Autodesk Inventor part; units mm, degrees
ref_plane "YZ Plane" through (0, 0, 0) normal (1, 0, 0) x (0, 1, 0)
ref_plane "XZ Plane" through (0, 0, 0) normal (0, 1, 0) x (-1, 0, 0)
ref_plane "XY Plane" through (0, 0, 0) normal (0, 0, 1) x (1, 0, 0)
sketch "Sketch1" plane through (0, 0, 0) normal (0, 0, 1) x (1, 0, 0)
  line L0 (-22.5, -30) -> (-22.5, 30)
  line L1 (-22.5, 30) -> (22.5, 30)
  line L2 (22.5, 30) -> (22.5, -30)
  line L3 (22.5, -30) -> (-22.5, -30)
  line L4 (-22.5, -30) -> (22.5, 30) construction
  line L5 (-22.5, 30) -> (22.5, -30) construction
  line L6 (-22.5, 30) -> (-22.5, 22.5)
  line L7 (0, -30) -> (0, -20)
  line L8 (0, -20) -> (-10, -20)
  line L9 (-10, -20) -> (10, -20)
  line L10 (-22.5, 22.5) -> (-10, -20)
  line L11 (22.5, 30) -> (22.5, 22.5)
  line L12 (22.5, 22.5) -> (10, -20)
  arc A0 (-10, -20) -> (10, -20) centre (0, -20) ccw
  point P0 (0, 0)
  dimension "d0" = 60
  dimension "d1" = 45
  dimension "d2" = 7.5
  dimension "d3" = 10
  dimension "d4" = 10
  dimension "d5" = 20
  dimension "d6" = 7.5
extrude "Extrusion1" add sketch "Sketch1" along normal blind 40 contours L0 L1 L2 L12 L9 L8 L10 | A0 L8 L7 | L7 L9 A0
sketch "Sketch2" plane through (0, 0, 0) normal (1, 0, 0) x (0, 1, 0)
  line L0 (30, 0) -> (30, 40)
  line L1 (30, 40) -> (30, 0)
  line L2 (-20, 0) -> (-30, 0)
  line L3 (30, 0) -> (-30, 0)
  line L4 (-30, 0) -> (-30, 1)
  line L5 (-30, 0) -> (-30, 40)
  line L6 (30, 40) -> (-30, 40)
  line L7 (-30, 40) -> (-30, 39)
  line L8 (-30, 39) -> (27.8612, 39)
  line L9 (30, 40) -> (22.5, 40)
  line L10 (-30, 1) -> (27.8612, 1)
  line L11 (27.8612, 1) -> (27.8612, 39)
  line L12 (-30, 39) -> (-30, 1)
  point P0 (0, 0)
  dimension "d9" = 1
  dimension "d10" = 1
extrude "Extrusion2" cut sketch "Sketch2" along normal through all both and the other way through all contours L5 L8 L11 L10
sketch "Sketch3" plane through (0, 0, 40) normal (0, 0, 1) x (1, 0, 0)
  arc A0 (-10, -20) -> (10, -20) centre (0, -20) ccw
  line L0 (10, -20) -> (22.5, 22.5)
  line L1 (22.5, 22.5) -> (22.5, 30)
  line L2 (22.5, 30) -> (-22.5, 30)
  line L3 (-22.5, 30) -> (-22.5, 22.5)
  line L4 (-22.5, 22.5) -> (-10, -20)
  circle A1 centre (0, -25.2901) radius 2.5
  point P0 (0, 0)
  dimension "d13" = 5
extrude "Extrusion3" cut sketch "Sketch3" against normal blind 40 contours A1
sketch "Sketch4" plane through (-22.5, 30, 0) normal (0, 1, 0) x (1, 0, 0)
  line L0 (45, -40) -> (0, -40)
  line L1 (45, 0) -> (0, 0)
  line L2 (0, -40) -> (45, 0) construction
  line L3 (0, 0) -> (0, -40)
  line L4 (0, 0) -> (45, -40) construction
  line L5 (0, -20) -> (45, -20) construction
  circle A0 centre (4.5627, -20) radius 2.5
  point P0 (22.5, 0)
  dimension "d16" = 5
extrude "Extrusion4" cut sketch "Sketch4" against normal blind 10
ref_plane "Work Plane1" through (0, 22.5, 0) normal (1, 0, 0) x (0, 0, -1)
mirror "Mirror1" about plane through (0, 22.5, 0) normal (1, 0, 0) of "Extrusion4"
properties part number "Thin Wheel Mount"
Check sheet for the modelled part. Datum: model origin and axes. Units: mm. A direction names the side the tool comes from. Give positions to 0.01 mm unless a question says otherwise; leave off trailing zeros. Order: outer loops, then holes, each group sorted by start corner. A loop starts at its lowest first (then second) coordinate and runs counter-clockwise, first axis right, second up. Notation, with made-up numbers: M 63,72 L 118,72 A22 cw 118,105 Z; hole C 41,32.25 d8. An arc over 180 degrees is marked long. Answer in a Markdown table with one row per item. Add a question column.
Q1. Gauge pin test, flat end, axial feed: pin 1 Ø5 at (x, z) = (3.5, 31) entering from -Y. Record the tip position at first contact, or that the pin passes through.
Q2. Release check for a two-part mould opening along X. For faces 1 (the flat face through (-22.5, 28.5, 19.9)), 2 (the flat face through (0, 30, 20)), 3 (the cylindrical face through (1.15, -27.51, 39.51)) record: released by +X, released by -X, zero draft, split by the parting line, or undercut.
Q3. Sectioned sample at C-C, the plane x = 19. Record the boundary of the cut face in (y, z).
Q4. Sectioned sample at B-B, the plane x = 0. Record the boundary of the cut face in (y, z), and give its area (3 significant figures).
Q5. Sectioned sample at D-D, the plane y = 11. Record the boundary of the cut face in (x, z), and give its area (3 significant figures).
Q6. Access from +Z, -Z, +X, -X, +Y, -Y to the whole of each face (thin tool, end or side, straight path). Record for faces 4 (the flat face through (0, 5, 39)), 5 (the flat face through (16.34, 1.55, 39.49)).
Q7. Thickness scan on L1, parallel to X at y = 28, z = 20; L2, parallel to Z at x = -7, y = -19.5; L3, parallel to Y at x = 0, z = 0.55. Record the ranges inside material, lowest first.
Q8. Sectioned sample at A-A, the plane z = 20. Record the boundary of the cut face in (x, y).
Verdict:
| question | item | result |
|---|---|---|
| 1 | pin 1 | y = 27.86 |
| 2 | face 1 | released by -X |
| 2 | face 2 | zero draft |
| 2 | face 3 | undercut |
| 3 | outline | M 10.6,0 L 30,0 L 30,17.74 L 27.86,17.74 L 27.86,1 L 10.6,1 Z; M 10.6,39 L 27.86,39 L 27.86,22.26 L 30,22.26 L 30,40 L 10.6,40 Z |
| 4 | outline | M -30,0 L -27.79,0 L -27.79,1 L -30,1 Z; M -30,39 L -27.79,39 L -27.79,40 L -30,40 Z; M -22.79,0 L 30,0 L 30,40 L -22.79,40 L -22.79,39 L 27.86,39 L 27.86,1 L -22.79,1 Z |
| 4 | area | 191 mm² |
| 5 | outline | M -19.12,0 L 19.12,0 L 19.12,1 L -19.12,1 Z; M -19.12,39 L 19.12,39 L 19.12,40 L -19.12,40 Z |
| 5 | area | 76.5 mm² |
| 6 | face 4 | +X, -X, -Y |
| 6 | face 5 | +Z, -Z, +X, -Y |
| 7 | L1 | -22.5 to -20.44, -15.44 to 15.44, 20.44 to 22.5 |
| 7 | L2 | 0 to 1, 39 to 40 |
| 7 | L3 | -30 to -27.79, -22.79 to 30 |
| 8 | outline | M -22.5,27.86 L -20.44,27.86 L -20.44,30 L -22.5,30 Z; M -15.44,27.86 L 15.44,27.86 L 15.44,30 L -15.44,30 Z; M 20.44,27.86 L 22.5,27.86 L 22.5,30 L 20.44,30 Z |
